```python
from build123d import *

# Parameters (mm, degrees)
F0_W     = 14.35
F0_H     = 90.5499906
F0_R     = 4
F0_R_2   = 1.8288
F0_W_2   = 8
F0_H_2   = 45.9749906
F1_DEPTH = 6.35
F2_SIZE  = 0.254
F3_W     = 7.9375
F3_H     = 7.9375
F4_DEPTH = 1.5875
F5_R     = 3.96874
F6_SIZE  = 0.508


# Not quite as in the source:
# - a fillet or chamfer is up to 0.001 mm smaller than in the source, because OpenCascade refuses the exact size


with BuildPart() as f1:
    # F0 (on Top) → F1 (new body)
    with BuildSketch(Plane.XY):
        Rectangle(F0_W, F0_H)
        with Locations((0, -38.0999953)):
            Circle(F0_R, mode=Mode.SUBTRACT)
        with Locations((0, -26.9562453)):
            Circle(F0_R_2, mode=Mode.SUBTRACT)
        Rectangle(F0_W_2, F0_H_2, mode=Mode.SUBTRACT)
        with Locations((0, 26.9562453)):
            Circle(F0_R_2, mode=Mode.SUBTRACT)
        with Locations((0, 38.0999953)):
            Circle(F0_R, mode=Mode.SUBTRACT)
    extrude(amount=F1_DEPTH)

    # F2
    f2_edges = [f1.edges().sort_by_distance(p)[0] for p in [
        (-4, 38.099995, 0),
        (-4, -38.099995, 0),
    ]]
    chamfer(f2_edges, length=F2_SIZE)

    # F3 (on face) → F4 (cut)
    with BuildSketch(Plane.XY.offset(6.35)):
        with Locations((0, 26.9562453)):
            Rectangle(F3_W, F3_H)
        with Locations((0, -26.9562453)):
            Rectangle(F3_W, F3_H)
    extrude(amount=-F4_DEPTH, mode=Mode.SUBTRACT)

    # F5 (radius 3.96875 in the source; OpenCascade refuses exactly that, so slightly less here)
    f5_edges = [f1.edges().sort_by_distance(p)[0] for p in [
        (-3.96875, -30.924995, 5.55625),
        (3.96875, -30.924995, 5.55625),
        (-3.96875, 30.924995, 5.55625),
        (3.96875, 30.924995, 5.55625),
    ]]
    fillet(f5_edges, radius=F5_R)

    # F6
    f6_edges = [f1.edges().sort_by_distance(p)[0] for p in [
        (-4, 38.099995, 6.35),
        (-4, -38.099995, 6.35),
    ]]
    chamfer(f6_edges, length=F6_SIZE)


solid = f1.part
```
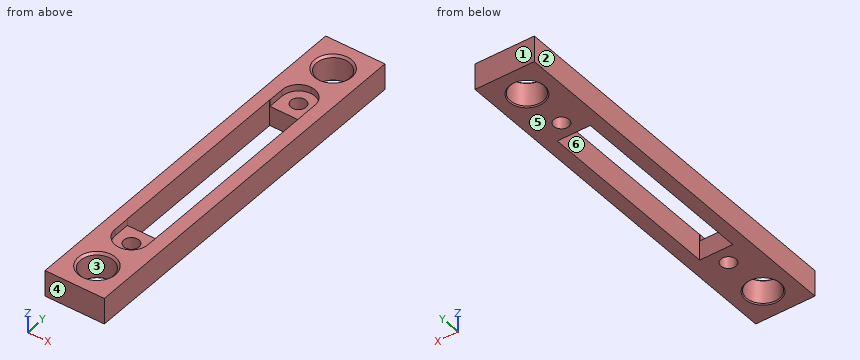
Source: CAD feature listing. Evaluate the final solid. Frame: model axes, mm. Face numbers are marked on the shaded views. A direction names the side the tool comes from. Round coordinates to 2 decimals unless told otherwise and drop trailing zeros. Loops run counter-clockwise (first coordinate to the right, second up) from the corner with the lowest first, then second, coordinate; pieces in that order, holes last.
(1) Section query A-A (z = 1.75). Output: boundary loops of the cut face in (x, y) (1 decimal).
From the geometry:
outline: (-7.2, -45.3) - (7.2, -45.3) - (7.2, 45.3) - (-7.2, 45.3) - close; hole circle Ø8 at (0, -38.1); hole (-4, -23) - (4, -23) - (4, 23) - (-4, 23) - close; hole circle Ø8 at (0, 38.1); hole circle Ø3.7 at (0, -27); hole circle Ø3.7 at (0, 27)
(2) Pull-direction query (Y, two-part tool) for the marked faces 1, 2, 3 and 4; classes: +Y half, -Y half, draft (parallel to the pull), parting line (faces both ways), or undercut.
From the geometry:
face 1: +Y half
face 2: draft
face 3: undercut
face 4: -Y half
(3) Access query for the marked faces 5 and 6. Directions: +Z, -Z, +X, -X, +Y, -Y. A direction counts if a zero-diameter tool reaches every point of the face in a straight line with its end or side. Return the directions, or none.
From the geometry:
face 5: -Z, +X, -X, +Y, -Y
face 6: +Z, -Z
(4) Contact query for a flat-ended pin moving along its axis: pin 1 Ø2 at (x, y) = (0, 26.96) entering from +Z. Output: stop coordinate, or through.
From the geometry:
pin 1: passes through
(5) Material intervals for probe 1 along Y at (x, z) = (0, 1.85) (1 decimal); probe 2 along Y at (x, z) = (0.25, 5) (3 decimals); probe 3 along X at (y, z) = (-1, 1.75) (3 decimals), sorted ascending.
From the geometry:
probe 1: y = -45.3 to -42.1, -34.1 to -28.8, -25.1 to -23, 23 to 25.1, 28.8 to 34.1, 42.1 to 45.3
probe 2: y = -45.275 to -42.092, -34.108 to -30.917, 30.917 to 34.108, 42.092 to 45.275
probe 3: x = -7.175 to -4, 4 to 7.175
